CAD build for the part. Positions are in the model's coordinates, mm. Give positions to 0.01 mm unless a question says otherwise; leave off trailing zeros. Loops run counter-clockwise (first coordinate to the right, second up) from the corner with the lowest first, then second, coordinate; pieces in that order, holes last. Notation, with made-up numbers: (-14.75, 37) -> (-4.75, 37) arc R17 cw to (-4.75, 51) -> close; hole circle Ø9 at (-38.5, 13.25). An arc over 180 degrees is marked (long way). Write each question's results on one line, items separated by ' | '. Start each with the question number.
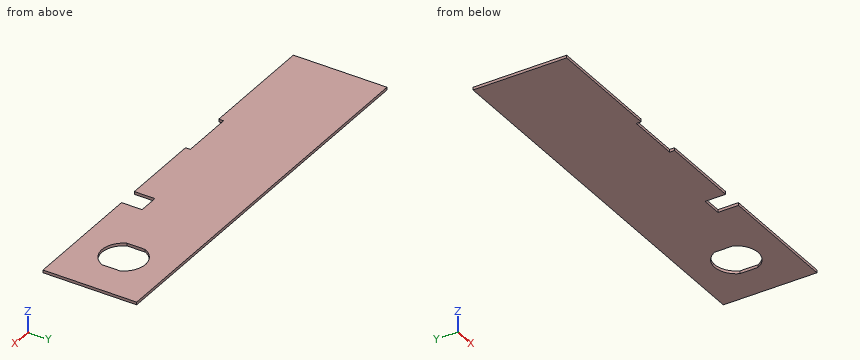
```python
from build123d import *

# Parameters (mm, degrees)
BOSS_EXTRUDE2_DEPTH = 1.778


with BuildPart() as part:
    # Sketch1 → Boss-Extrude2 (new body)
    with BuildSketch(Plane.XY):
        Polygon((109.4486, 0), (161.29, 0), (161.29, 13.1699), (174.3202, 13.1699), (174.3202, 0), (254, 0), (254, 60.071), (0, 60.071), (0, 0), (75.6158, 0), (75.6158, 3.1115), (109.4486, 3.1115), align=None)
        with BuildLine():
            Line((232.41, 35.855371133), (232.41, 24.215628867))
            ThreePointArc((232.41, 24.215628867), (219.71, 16.0655), (207.01, 24.215628867))
            Line((207.01, 24.215628867), (207.01, 35.855371133))
            ThreePointArc((207.01, 35.855371133), (219.71, 44.0055), (232.41, 35.855371133))
        make_face(mode=Mode.SUBTRACT)
    extrude(amount=BOSS_EXTRUDE2_DEPTH)


solid = part.part
```
Q1. Saw through at C-C, the plane y = 38.5. List the corners of the cut face in (x, z).
Q2. Saw through at A-A, the plane y = 27. List the corners of the cut face in (x, z), then the cut area to 3 significant figures.
Q3. Saw through at B-B, the plane z = 0.6. List the corners of the cut face in (x, y), then the cut area to 3 significant figures.
Q4. Wall check: L1, parallel to X at y = 6, z = 0.95; L2, parallel to Y at x = 88, z = 1.05; L3, parallel to X at y = 30, z = 0.95. Give the ranges that are in metal, low to high.
Q5. Drop flat-ended pins along their axis: pin 1 (1.5 mm diameter, centred on x = 97, y = 43, fed in from -Z); pin 2 (0.5 mm diameter, centred on x = 169.5, z = 1, fed in from -Y). Give the stop position or say it passes through.
Answer block:
1) outline: (0, 0) -> (208.6, 0) -> (208.6, 1.78) -> (0, 1.78) -> close; (230.82, 0) -> (254, 0) -> (254, 1.78) -> (230.82, 1.78) -> close
2) outline: (0, 0) -> (207.01, 0) -> (207.01, 1.78) -> (0, 1.78) -> close; (232.41, 0) -> (254, 0) -> (254, 1.78) -> (232.41, 1.78) -> close | area: 406 mm2
3) outline: (0, 0) -> (75.62, 0) -> (75.62, 3.11) -> (109.45, 3.11) -> (109.45, 0) -> (161.29, 0) -> (161.29, 13.17) -> (174.32, 13.17) -> (174.32, 0) -> (254, 0) -> (254, 60.07) -> (0, 60.07) -> close; hole (207.01, 24.22) arc R13.97 ccw to (232.41, 24.22) -> (232.41, 35.86) arc R13.97 ccw to (207.01, 35.86) -> close | area: 14,400 mm2
4) L1: x = 0 to 161.29, 174.32 to 254 | L2: y = 3.11 to 60.07 | L3: x = 0 to 207.01, 232.41 to 254
5) pin 1: stops at z = 0 | pin 2: stops at y = 13.17
